from build123d import *

# Parameters (mm, degrees)
SKETCH1_R           = 4.1
BOSS_EXTRUDE1_DEPTH = 4
SKETCH2_R           = 4.1
BOSS_EXTRUDE2_DEPTH = 0.8
SKETCH3_R           = 3.5
CUT_EXTRUDE1_DEPTH  = 1.8


with BuildPart() as part:
    # Sketch1 → Boss-Extrude1 (new body)
    with BuildSketch(Plane(origin=(0, 0, 0), x_dir=(1, 0, 0), z_dir=(0, 1, 0))):
        with BuildLine():
            ThreePointArc((-6.55, 0), (0, -6.55), (6.55, 0))
            Line((6.55, 0), (6.55, 17))
            ThreePointArc((6.55, 17), (0, 23.55), (-6.55, 17))
            Line((-6.55, 17), (-6.55, 0))
        make_face()
        Circle(SKETCH1_R, mode=Mode.SUBTRACT)
        with BuildLine():
            Line((-1.55, 8.1), (-1.55, 17))
            ThreePointArc((-1.55, 17), (0, 18.55), (1.55, 17))
            Line((1.55, 17), (1.55, 8.1))
            ThreePointArc((1.55, 8.1), (0, 6.55), (-1.55, 8.1))
        make_face(mode=Mode.SUBTRACT)
    extrude(amount=BOSS_EXTRUDE1_DEPTH)

    # Sketch2 → Boss-Extrude2 (add)
    with BuildSketch(Plane(origin=(0, 0, 0), x_dir=(1, 0, 0), z_dir=(0, 1, 0))):
        Circle(SKETCH2_R)
    extrude(amount=BOSS_EXTRUDE2_DEPTH)

    # Sketch3 → Cut-Extrude1 (cut, through all)
    with BuildSketch(Plane(origin=(0, 0.8, 0), x_dir=(1, 0, 0), z_dir=(0, 1, 0))):
        Circle(SKETCH3_R)
    extrude(amount=-CUT_EXTRUDE1_DEPTH, mode=Mode.SUBTRACT)


solid = part.part
Geometry check sheet. Reference: the model listing, model coordinates, mm. A direction names the side the tool comes from. Give positions to 0.01 mm unless a question says otherwise; leave off trailing zeros. Loops run counter-clockwise (first coordinate to the right, second up) from the corner with the lowest first, then second, coordinate; pieces in that order, holes last. Notation, with made-up numbers: (-31.5, 17.5) -> (-26.5, 17.5) arc R26 cw to (-26.5, 44.5) -> close; hole circle Ø8 at (79.25, -19). An arc over 180 degrees is marked (long way). Answer in a Markdown table with one row per item. Add a question column.
1) Draft check along Z on faces 1 (the face through (6.55, 2, -8)), 2 (the face through (0.14, 1.97, -23.55)), 3 (the face through (1.55, 2, -13)). Enter one of: pulls with the +Z half, pulls with the -Z half, needs draft (parallel to the pull), parting line crosses it, or undercut.
2) Gauge pin test, flat ends, axial feed: P1, Ø2.5, axis at x = 2, z = -1.5, coming from the +Y side; P2, Ø2, axis at x = 5, y = 3, coming from the +Z side; P3, Ø5, axis at x = 0, z = 0, coming from the -Y side; P4, Ø1, axis at x = 1.5, y = 3, coming from the +Z side. Record the tip position at first contact, or that the pin passes through.
3) Cross-section at A-A on z = -9. Record the boundary of the cut face in (x, y).
4) Set-up check for faces 4 (the face through (3, 4, -9)), 5 (the face through (-0.03, 1.97, -18.55)), 6 (the face through (-0.534, 2.378, -4.065)): record each of +Z, -Z, +X, -X, +Y, -Y from which the full face is reachable in a straight line by a thin tool's end or side.
5) Cross-section at D-D on y = 0.5. Record the boundary of the cut face in (x, z), and give its area (3 significant figures).
6) Cross-section at B-B on x = 0. Record the boundary of the cut face in (y, z).
7) Cross-section at C-C on y = 1.9. Record the boundary of the cut face in (x, z).
8) Material ranges on probe 1 along Z at (x, y) = (0, 0.4); probe 2 along Z at (x, y) = (0, 2); probe 3 along X at (y, z) = (2.4, -8.5), recorded low to high. Write a range as from..to.
Outcome:
| question | item | result |
|---|---|---|
| 1 | face 1 | needs draft |
| 1 | face 2 | pulls with the -Z half |
| 1 | face 3 | undercut |
| 2 | P1 | stops at y = 0.8 |
| 2 | P2 | stops at z = 5.19 |
| 2 | P3 | passes through |
| 2 | P4 | stops at z = 6.47 |
| 3 | outline | (-6.55, 0) -> (-1.55, 0) -> (-1.55, 4) -> (-6.55, 4) -> close; (1.55, 0) -> (6.55, 0) -> (6.55, 4) -> (1.55, 4) -> close |
| 4 | face 4 | +Z, -Z, +X, -X, +Y |
| 4 | face 5 | +Y, -Y |
| 4 | face 6 | +Y |
| 5 | outline | (-6.55, -17) arc R6.55 ccw to (6.55, -17) -> (6.55, 0) arc R6.55 ccw to (-6.55, 0) -> close; hole circle Ø7 at (0, 0); hole (-1.55, -17) arc R1.55 ccw to (1.55, -17) -> (1.55, -8.1) arc R1.55 ccw to (-1.55, -8.1) -> close |
| 5 | area | 284 mm^2 |
| 6 | outline | (0, -23.55) -> (4, -23.55) -> (4, -18.55) -> (0, -18.55) -> close; (0, -6.55) -> (4, -6.55) -> (4, -4.1) -> (0.8, -4.1) -> (0.8, -3.5) -> (0, -3.5) -> close; (0, 3.5) -> (0.8, 3.5) -> (0.8, 4.1) -> (4, 4.1) -> (4, 6.55) -> (0, 6.55) -> close |
| 7 | outline | (-6.55, -17) arc R6.55 ccw to (6.55, -17) -> (6.55, 0) arc R6.55 ccw to (-6.55, 0) -> close; hole circle Ø8.2 at (0, 0); hole (-1.55, -17) arc R1.55 ccw to (1.55, -17) -> (1.55, -8.1) arc R1.55 ccw to (-1.55, -8.1) -> close |
| 8 | probe 1 | z = -23.55..-18.55, -6.55..-3.5, 3.5..6.55 |
| 8 | probe 2 | z = -23.55..-18.55, -6.55..-4.1, 4.1..6.55 |
| 8 | probe 3 | x = -6.55..-1.55, 1.55..6.55 |
